```python
from build123d import *

# Parameters (mm, degrees)
SKETCH1_W           = 25.4
SKETCH1_H           = 12.7
BOSS_EXTRUDE1_DEPTH = 381
SKETCH2_R           = 6.35
CUT_EXTRUDE1_DEPTH  = 383.056867495
SKETCH3_W           = 25.4
SKETCH3_H           = 58.414427835
CUT_EXTRUDE2_DEPTH  = 6.35


with BuildPart() as part:
    # Sketch1 → Boss-Extrude1 (new body)
    with BuildSketch(Plane(origin=(0, 0, 0), x_dir=(1, 0, 0), z_dir=(0, 1, 0))):
        with Locations((12.7, 6.35)):
            Rectangle(SKETCH1_W, SKETCH1_H)
    extrude(amount=BOSS_EXTRUDE1_DEPTH)

    # Sketch2 → Cut-Extrude1 (cut, through all)
    with BuildSketch(Plane.XY):
        with Locations(Location((12.7, 330.2, 0), (0, 0, 180))):
            Circle(SKETCH2_R)
    extrude(amount=-CUT_EXTRUDE1_DEPTH, mode=Mode.SUBTRACT)

    # Sketch3 → Cut-Extrude2 (cut)
    with BuildSketch(Plane.XY):
        with Locations((12.7, 329.619745597)):
            Rectangle(SKETCH3_W, SKETCH3_H)
    extrude(amount=-CUT_EXTRUDE2_DEPTH, mode=Mode.SUBTRACT)


solid = part.part
```
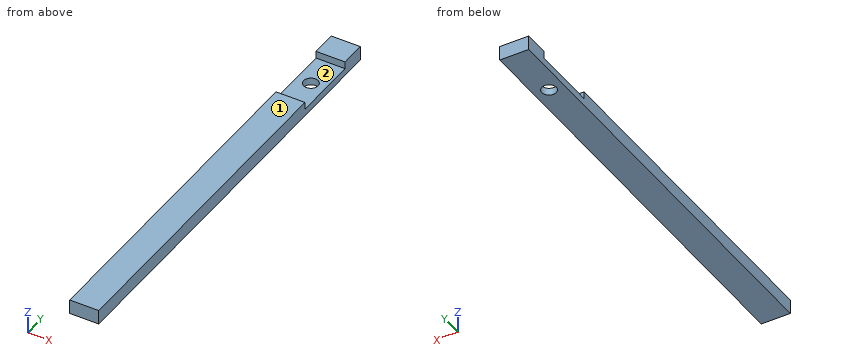
The listing builds one solid part. Answer for the finished solid, in the listing's coordinates (mm). Face numbers are marked on the shaded views. Coordinates: 2 decimals unless noted, no trailing zeros. Loops run counter-clockwise (first coordinate to the right, second up) from the corner with the lowest first, then second, coordinate; pieces in that order, holes last. Notation, with made-up numbers: M -10.5,85.5 L 28.5,85.5 A30 cw 28.5,118.5 Z; hole C 69,-27 d11. An arc over 180 degrees is marked long. Answer as CSV lines item,"result". Start each with the question number.
(1) The part is cut by section A-A (x = 12.7). Give the vertices of the cut face in (y, z), and give its area (3 significant figures).
(2) The part is cut by section B-B (y = 330.2). Give the vertices of the cut face in (x, z), and give its area (3 significant figures).
(3) Find the intervals of material crossed by L1, parallel to Y at x = 18.25, z = -2.25; L2, parallel to Y at x = 12.7, z = -7.75; L3, parallel to X at y = 330.2, z = -10.75, in increasing order. Write a range as [from, to].
(4) Given pin 1 (14.5 mm diameter, centred on x = 12.7, y = 330.2, fed in from +Z), flat-ended and moving along its own axis, determine where the tip first touches the part or whether it passes through.
(5) The mould has two halves that part along Y. Classify the marked faces 1 and 2: pulls with the +Y half, pulls with the -Y half, needs draft (parallel to the pull), parting line crosses it, or undercut.
Determined:
1,outline,"M 0,-12.7 L 323.85,-12.7 L 323.85,-6.35 L 300.41,-6.35 L 300.41,0 L 0,0 Z; M 336.55,-12.7 L 381,-12.7 L 381,0 L 358.83,0 L 358.83,-6.35 L 336.55,-6.35 Z"
1,area,"4,390 mm2"
2,outline,"M 0,-12.7 L 6.35,-12.7 L 6.35,-6.35 L 0,-6.35 Z; M 19.05,-12.7 L 25.4,-12.7 L 25.4,-6.35 L 19.05,-6.35 Z"
2,area,"80.6 mm2"
3,L1,"[0, 300.41], [358.83, 381]"
3,L2,"[0, 323.85], [336.55, 381]"
3,L3,"[0, 6.35], [19.05, 25.4]"
4,pin 1,"z = -6.35"
5,face 1,"needs draft"
5,face 2,"undercut"
